The model under review builds one solid part; all positions refer to its coordinate system, in mm. Coordinates: 2 decimals unless noted, no trailing zeros. Order: outer loops, then holes, each group sorted by start corner. A loop starts at its lowest first (then second) coordinate and runs counter-clockwise, first axis right, second up. Notation, with made-up numbers: (-18.75, -29.75) -> (-6.75, -29.75) arc R4 cw to (-6.75, -22.75) -> close; hole circle Ø6 at (18.25, 67). An arc over 180 degrees is marked (long way). Use one line per item in the form item = value.
from build123d import *

# Parameters (mm, degrees)
SKETCH_1_R          = 17
EXTRUDE_1_DEPTH     = 8
SKETCH_2_R          = 1.65
CUT_EXTRUDE_1_DEPTH = 20
FILLET_1_R          = 1


with BuildPart() as part:
    # Эскиз1 → Бобышка-Вытянуть1 (new body)
    with BuildSketch(Plane(origin=(0, 0, 0), x_dir=(1, 0, 0), z_dir=(0, 1, 0))):
        with Locations(Location((0, 0, 0), (0, 0, 270))):
            Circle(SKETCH_1_R)
    extrude(amount=EXTRUDE_1_DEPTH)

    # Эскиз2 → Вырез-Вытянуть1 (cut)
    with BuildSketch(Plane(origin=(0, 8, 0), x_dir=(1, 0, 0), z_dir=(0, 1, 0))):
        with Locations(Location((0, 13.5, 0), (0, 0, 270))):
            Circle(SKETCH_2_R)
        with Locations(Location((11.691342951, -6.75, 0), (0, 0, 270))):
            Circle(SKETCH_2_R)
        with Locations(Location((-11.691342951, -6.75, 0), (0, 0, 270))):
            Circle(SKETCH_2_R)
    extrude(amount=-CUT_EXTRUDE_1_DEPTH, mode=Mode.SUBTRACT)

    # Скругление1
    fillet_1_edges = [part.edges().sort_by_distance(p)[0] for p in [
        (0, 8, -17),
    ]]
    fillet(fillet_1_edges, radius=FILLET_1_R)


solid = part.part
Item 1: We need section A-A (z = 6.75). State how many separate pieces and enclosed holes the cut face has, plus the area to 3 significant figures.
Results found:
separate_pieces = 3
enclosed_holes = 0
area = 196 mm²
Item 2: We need section B-B (y = 5.25). Write out the cut boundary in (x, z), plus the area to 3 significant figures.
Results found:
outline = circle Ø34 at (0, 0); hole circle Ø3.3 at (-11.69, 6.75); hole circle Ø3.3 at (0, -13.5); hole circle Ø3.3 at (11.69, 6.75)
area = 882 mm²
Item 3: Draft analysis for pull direction X (two halves, no side actions). For faces 1 (the face through (0, 0, 0)), 2 (the face through (-12.695, 4.056, 5.441)), 3 (the face through (16.855, 3.451, -2.213)), state which applies: released by +X, released by -X, zero draft, split by the parting line, or undercut.
Results found:
face_1 = zero draft
face_2 = undercut
face_3 = split by the parting line
Item 4: Clearance check with flat-ended pins moving along their axes: pin 1 (3 mm diameter, centred on x = 3.5, y = 4, fed in from -Z); pin 2 (2 mm diameter, centred on x = 7.5, y = 6.5, fed in from -Z); pin 3 (2 mm diameter, centred on x = 12.5, y = 5.5, fed in from -Z). State where each tip first meets the part, or that it passes through.
Results found:
pin_1 = -16.88
pin_2 = -15.71
pin_3 = -12.52
Item 5: To check wall thickness, follow L1, parallel to X at y = 6.25, z = 8; L2, parallel to Y at x = -9.5, z = -13; L3, parallel to X at y = 4, z = 6.75. State the ranges of each line that lie inside material, in increasing order. Write a range as from..to.
Results found:
L1 = -15..-12.77, -10.61..10.61, 12.77..15
L2 = 0..7.99
L3 = -15.6..-13.34, -10.04..10.04, 13.34..15.6
